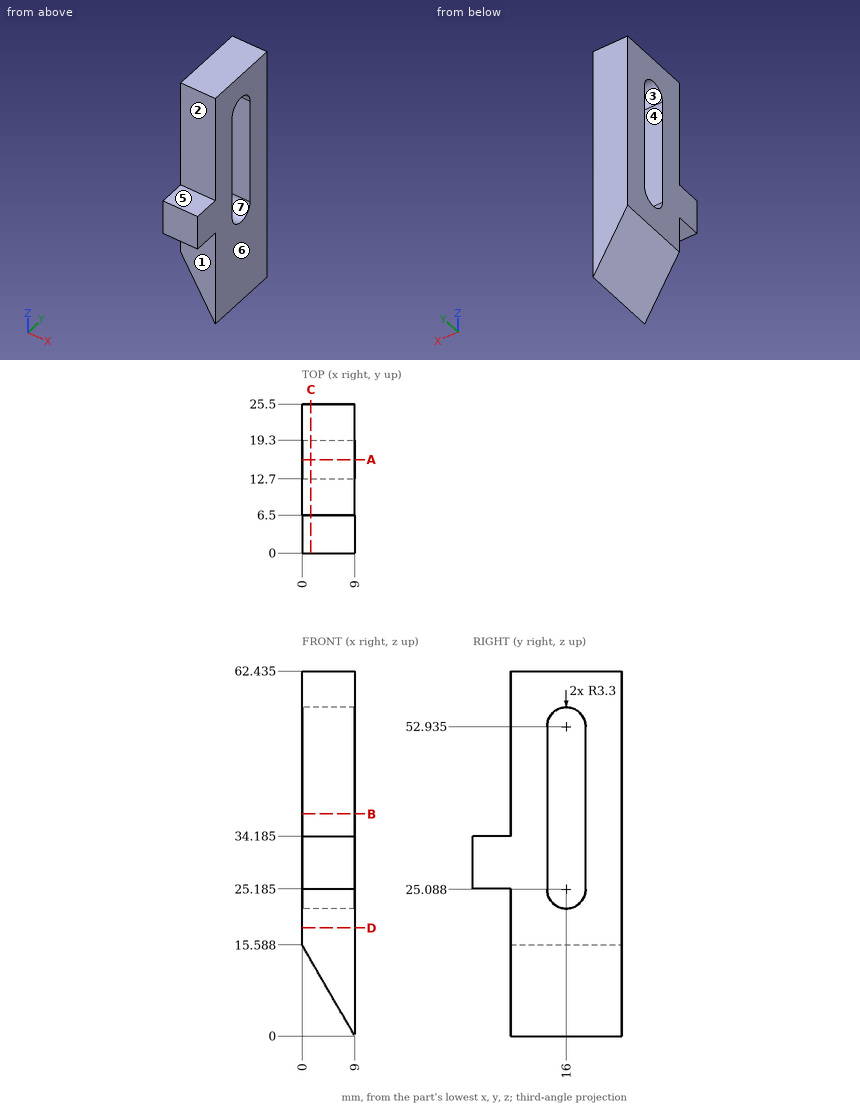
Answer from the drawing. Dimensions are ordinates in mm from the lowest x, y and z of the part. A direction names the side the tool comes from. Give positions to 0.01 mm unless a question says otherwise; leave off trailing zeros. Loops run counter-clockwise (first coordinate to the right, second up) from the corner with the lowest first, then second, coordinate; pieces in that order, holes last.
Item 1: For the marked faces 1, 2 and 3, determine the directions among +Z, -Z, +X, -X, +Y, -Y from which every point of the face is accessible in a straight line to the end or side of a thin tool.
Item 2: The part is cut by section A-A (y = 16). Write down the section's boundary in (x, z) (1 decimal).
Item 3: Find the intervals of material crossed by line 1 along Y through (x, z) = (3, 38); line 2 along Y through (x, z) = (8, 59); line 3 along Z through (x, y) = (1.75, 2.75) (1 decimal), in increasing order.
Item 4: The part is cut by section D-D (z = 18.5). Write down the section's boundary in (x, y), and give its area (3 significant figures).
Item 5: The part is cut by section C-C (x = 1.5). Write down the section's boundary in (y, z) (1 decimal).
Item 6: The mould has two halves that part along Z. Classify the marked faces 4, 5, 6 and 7: released by +Z, released by -Z, zero draft, split by the parting line, or undercut.
Item 7: Each of these flat-tipped pins is pushed along its axis until it touches: pin 1 Ø2.5 at (x, z) = (3, 36) entering from -Y; pin 2 Ø3 at (x, y) = (3.5, 4.5) entering from +Z (1 decimal). Where does it stop, or does it pass through?
Item 8: The part is cut by section B-B (z = 38). Write down the section's boundary in (x, y).
Taken from the geometry:
1. face 1: -Z, +X, -X, -Y
1. face 2: +Z, +X, -X, -Y
1. face 3: +X, -X
2. outline: (0, 15.6) - (9, 0) - (9, 21.8) - (0, 21.8) - close; (0, 56.2) - (9, 56.2) - (9, 62.4) - (0, 62.4) - close
3. line 1: y = 6.5 to 12.7, 19.3 to 25.5
3. line 2: y = 6.5 to 25.5
3. line 3: z = 25.2 to 34.2
4. outline: (0, 6.5) - (9, 6.5) - (9, 25.5) - (0, 25.5) - close
4. area: 171 mm2
5. outline: (0, 25.2) - (6.5, 25.2) - (6.5, 13) - (25.5, 13) - (25.5, 62.4) - (6.5, 62.4) - (6.5, 34.2) - (0, 34.2) - close; hole (12.7, 25.1) arc R3.3 ccw to (19.3, 25.1) - (19.3, 52.9) arc R3.3 ccw to (12.7, 52.9) - close
6. face 4: undercut
6. face 5: released by +Z
6. face 6: zero draft
6. face 7: undercut
7. pin 1: stops at y = 6.5
7. pin 2: stops at z = 34.2
8. outline: (0, 6.5) - (9, 6.5) - (9, 12.7) - (0, 12.7) - close; (0, 19.3) - (9, 19.3) - (9, 25.5) - (0, 25.5) - close
